Autodesk Inventor part; units mm, degrees
ref_plane "YZ Plane" through (0, 0, 0) normal (1, 0, 0) x (0, 1, 0)
ref_plane "XZ Plane" through (0, 0, 0) normal (0, 1, 0) x (-1, 0, 0)
ref_plane "XY Plane" through (0, 0, 0) normal (0, 0, 1) x (1, 0, 0)
sketch "Sketch1" plane through (0, 0, 0) normal (0, 1, 0) x (-1, 0, 0)
  line L0 (19, 19) -> (-19, 19)
  line L1 (-19, 19) -> (-19, -19)
  line L2 (-19, -19) -> (19, -19)
  line L3 (19, -19) -> (19, 19)
  line L4 (19, 19) -> (-19, -19) construction
  line L5 (-19, 19) -> (19, -19) construction
  line L6 (15, 15) -> (-15, 15) construction
  line L7 (-15, 15) -> (-15, -15) construction
  line L8 (-15, -15) -> (15, -15) construction
  line L9 (15, -15) -> (15, 15) construction
  line L10 (15, 15) -> (-15, -15) construction
  line L11 (-15, 15) -> (15, -15) construction
  circle A0 centre (15, 15) radius 1.25
  circle A1 centre (15, -15) radius 1.25
  circle A2 centre (-15, -15) radius 1.25
  circle A3 centre (-15, 15) radius 1.25
  point P0 (0, 0)
  dimension "d0" = 38
  dimension "d1" = 38
  dimension "d2" = 30
  dimension "d3" = 30
  dimension "d4" = 2.5
  dimension "d5" = 2.5
  dimension "d6" = 2.5
  dimension "d7" = 2.5
extrude "Extrusion1" add sketch "Sketch1" along normal blind 1
fillet "Fillet1" radius 3 4 edges at (19, 0.5, 19) (19, 0.5, -19) (-19, 0.5, -19) (-19, 0.5, 19)
sketch "Sketch2" plane through (0, 0, 0) normal (1, 0, 0) x (0, 1, 0)
  line L0 (43.1895, 0) -> (0.9392, 0)
  line L1 (1, 16) -> (1, -16) construction
  line L2 (0, 16) -> (0, -16)
  line L3 (0.9392, 0) -> (1, -14.9999)
  line L4 (1, -16) -> (1, 16)
  line L5 (1, -14.9999) -> (11.1999, -14.9585)
  line L6 (11.1999, -14.9585) -> (11.1898, -12.4586)
  line L7 (11.1898, -12.4586) -> (43.1895, -12.3289)
  line L8 (43.1895, -12.3289) -> (43.1895, 0)
  point P0 (0, 0)
  dimension "d16" = 15
  dimension "d17" = 10.2
  dimension "d18" = 2.5
  dimension "d19" = 32
revolve "Revolution1" add sketch "Sketch2" angle 360 about axis through (0, 43.1895, 0) along (0, -1, 0)
sketch "Sketch3" plane through (0, 43.1895, 0) normal (0, 1, 0) x (1, 0, 0)
  circle A0 centre (0, 0) radius 11.5
  dimension "d20" = 23
extrude "Extrusion2" cut sketch "Sketch3" against normal blind 2
sketch "Sketch4" plane through (0, 41.1895, 0) normal (0, 1, 0) x (1, 0, 0)
  circle A0 centre (0, 0) radius 8
  dimension "d23" = 16
extrude "Extrusion3" cut sketch "Sketch4" against normal blind 1
sketch "Sketch5" plane through (0, 0, 0) normal (0, -1, 0) x (1, 0, 0)
  circle A0 centre (-12, 0) radius 2.5
  line L0 (-19, -16) -> (-19, 16)
  circle A1 centre (12, 0) radius 2.5
  line L1 (19, 16) -> (19, -16)
  point P0 (0, 0)
  dimension "d26" = 5
  dimension "d27" = 7
  dimension "d28" = 5
  dimension "d29" = 7
extrude "Extrusion4" add sketch "Sketch5" along normal blind 3
sketch "Sketch6" plane through (0, 0, 0) normal (0, -1, 0) x (1, 0, 0)
  line L0 (-16, 19) -> (16, 19)
  line L1 (-10, 13.5) -> (10, 13.5)
  line L2 (10, 13.5) -> (10, 19)
  line L3 (10, 19) -> (-10, 19)
  line L4 (-10, 19) -> (-10, 13.5)
  line L5 (-10, 13.5) -> (10, 19) construction
  line L6 (10, 13.5) -> (-10, 19) construction
  point P0 (0, 0)
  point P1 (0, 16.25)
  dimension "d32" = 20
  dimension "d33" = 5.5
extrude "Extrusion5" add sketch "Sketch6" along normal blind 2
properties part number "camera"
Check sheet for the modelled part. Datum: model origin and axes. Units: mm. A direction names the side the tool comes from. Give positions to 0.01 mm unless a question says otherwise; leave off trailing zeros. Order: outer loops, then holes, each group sorted by start corner. A loop starts at its lowest first (then second) coordinate and runs counter-clockwise, first axis right, second up. Notation, with made-up numbers: (-22, 10.5) -> (-10, 10.5) arc R31 cw to (-10, 49.5) -> close; hole circle Ø8 at (75, 35). An arc over 180 degrees is marked (long way). Use CSV: the item, a comma, the result in double quotes. Start each with the question number.
1) Set-up check for faces 1 (the face through (10, -1, 16)), 2 (the face through (9.5, -1.5, -0.1)), 3 (the face through (0, 40.19, 0)): record each of +Z, -Z, +X, -X, +Y, -Y from which the full face is reachable in a straight line by a thin tool's end or side.
2) Go/stop test with flat-tipped pins: P1, Ø4, axis at x = 15, z = -15, coming from the +Y side; P2, Ø3, axis at x = -1.5, z = 16, coming from the -Y side; P3, Ø2, axis at x = 3.5, y = 33, coming from the +Z side (3 decimals). Record where each tip stops, or that it passes through.
3) Sectioned sample at A-A, the plane y = 32.5. Record the boundary of the cut face in (x, z).
4) Mould release check, pull along Z, two halves, no side actions. Record for faces 4 (the face through (-14.079, 0.493, -15.845)), 5 (the face through (12, -3, 0)), 6 (the face through (-7.542, 26.966, 9.836)): released by +Z, released by -Z, zero draft, split by the parting line, or undercut.
5) Material ranges on line 1 (Z direction, x = 15, y = 0.45); line 2 (X direction, y = 42.6, z = 0); line 3 (Y direction, x = 14, z = 0.5), recorded low to high. Write a range as from..to.
6) Sectioned sample at B-B, the plane y = 37.5. Record the boundary of the cut face in (x, z).
Recorded:
1,face 1,"+Z, +X, -Y"
1,face 2,"-Y"
1,face 3,"+Y"
2,P1,"y = 1"
2,P2,"y = -2"
2,P3,"z = 12.115"
3,outline,"circle Ø24.74 at (0, 0)"
4,face 4,"undercut"
4,face 5,"zero draft"
4,face 6,"split by the parting line"
5,line 1,"-19..-16.25, -13.75..13.75, 16.25..19"
5,line 2,"-12.33..-11.5, 11.5..12.33"
5,line 3,"-3..11.2"
6,outline,"circle Ø24.7 at (0, 0)"
